The model under review builds one solid part; all positions refer to its coordinate system, in mm. A direction names the side the tool comes from. Coordinates: 2 decimals unless noted, no trailing zeros. Loops run counter-clockwise (first coordinate to the right, second up) from the corner with the lowest first, then second, coordinate; pieces in that order, holes last. Notation, with made-up numbers: M 69.5,89.5 L 111.5,89.5 A22 cw 111.5,111.5 Z; hole C -2.75,47 d10. An arc over 180 degrees is marked long. Use one line per item in the form item = value.
Autodesk Fusion 360 part; units mm, degrees
sketch "スケッチ1" plane through (0, 0, 0) normal (0, 0, 1) x (1, 0, 0)
  circle A0 centre (0, 0) radius 10
  line L0 (0, 10) -> (12, 10)
  line L1 (12, 10) -> (12, 20)
  line L2 (12, 20) -> (27, 20)
  line L3 (27, 20) -> (27, 13)
  line L4 (27, 13) -> (23, 13)
  line L5 (23, 13) -> (23, 16)
  line L6 (23, 16) -> (19, 16)
  line L7 (19, 16) -> (19, -22)
  line L8 (19, -22) -> (12, -22)
  line L9 (12, -22) -> (12, -10)
  line L10 (12, -10) -> (0, -10)
  line L11 (0, -7) -> (0, 7)
  line L12 (19, -7) -> (14, -7)
  line L13 (14, -7) -> (14, 7)
  line L14 (14, 7) -> (19, 7)
  point P0 (14, 0)
  dimension "d1" = 20
  dimension "d2" = 12
  dimension "d4" = 4
  dimension "d5" = 4
  dimension "d6" = 7
  dimension "d8" = 4
  dimension "d9" = 3
  dimension "d19" = 14
  dimension "d29" = 13
  dimension "d30" = 22
  dimension "d31" = 5
  dimension "d32" = 14
extrude "押し出し1" add sketch "スケッチ1" along normal blind 8 contours A0 | A0 L0 L1 L2 L3 L4 L5 L6 L7 L8 L9 L10 L12 L13 L14
sketch "スケッチ2" plane through (0, 0, 8) normal (0, 0, 1) x (-1, 0, 0)
  arc A0 (0, -10) -> (0, 10) centre (0, 0) ccw
  line L0 (0, 10) -> (-12, 10)
  line L1 (-12, 10) -> (-12, 22)
  line L2 (-12, 22) -> (-19, 22)
  line L3 (-19, -7) -> (-19, -16)
  line L4 (-19, -16) -> (-23, -16)
  line L5 (-23, -16) -> (-23, -13)
  line L6 (-23, -13) -> (-27, -13)
  line L7 (-27, -13) -> (-27, -20)
  line L8 (-27, -20) -> (-12, -20)
  line L9 (-12, -20) -> (-12, -10)
  line L10 (-12, -10) -> (0, -10)
  circle A1 centre (0, 0) radius 10
  line L11 (-19, 7) -> (-14, 7)
  line L12 (-14, 7) -> (-14, -7)
  line L13 (-14, -7) -> (-19, -7)
  line L14 (-19, 22) -> (-19, 7)
extrude "押し出し2" add sketch "スケッチ2" along normal blind 1.5 contours A0 A1
hole "穴1" at (0, 7, 0) at (0, -7, 0) direction (0, 0, 1) diameter 3.2 end through all
hole "穴3" at (0, 0, 0) direction (0, 0, 1) diameter 8 end through all
sketch "スケッチ3" plane through (0, -10, 0) normal (0, -1, 0) x (1, 0, 0)
  line L0 (0, 0) -> (12, 0)
  line L1 (12, 0) -> (12, 8)
  line L2 (12, 8) -> (0, 8)
  line L3 (0, 8) -> (0, 0)
  line L4 (10, 0) -> (4, 4.5)
  line L5 (4, 4.5) -> (-15, 4.5)
  line L6 (-15, 4.5) -> (-15, 0)
  line L7 (-15, 0) -> (10, 0)
  dimension "d20" = 10
  dimension "d21" = 15
  dimension "d22" = 6
  dimension "d23" = 4.5
extrude "押し出し3" cut sketch "スケッチ3" against normal through all contours L0 L3 L4 L5 L7 | L3 L5 L6 L7
sketch "スケッチ4" plane through (19, 0, 0) normal (1, 0, 0) x (0, 1, 0)
  line L0 (-22, 0) -> (-7, 0)
  line L1 (16, 0) -> (16, 8)
  line L2 (-7, 8) -> (-22, 8)
  line L3 (-22, 8) -> (-22, 0)
  line L4 (-22, 4) -> (-18, 4)
  line L5 (-7, 0) -> (-7, 8)
  line L6 (7, 0) -> (16, 0)
  line L7 (16, 8) -> (7, 8)
  line L8 (7, 8) -> (7, 0)
  dimension "d25" = 4
hole "穴2" at (19, -18, 4) direction (-1, 0, 0) diameter 3 depth 11 tip angle 118
thread "ねじ1"
chamfer "面取り1" distance 1 angle 45 1 edges at (23, 13, 4)
fillet "フィレット1" radius 4 4 edges at (12, 10, 4) (12, -10, 4) (14, -7, 4) (14, 7, 4)
1. Add section D-D (y = 17). State the section outline as (x, z) points.
Response values:
outline = M 12,0 L 27,0 L 27,8 L 12,8 Z
2. Insertion check: P1, Ø0.6, axis at y = 14.5, z = 4.5, coming from the -X side; P2, Ø8, axis at x = 15.5, y = -6, coming from the +Z side; P3, Ø5, axis at x = -4, z = 6.5, coming from the +Y side; P4, Ø3.5, axis at x = 0, y = -7, coming from the +Z side. Each pin has a flat end and moves straight along its axis. Give the tip position at first contact, or say it passes through.
Response values:
P1 = 12
P2 = 8
P3 = 9.89
P4 = 9.5
3. Wall thickness on line 1 along Y through (x, z) = (0, 6.35); line 2 along Z through (x, y) = (13.5, -18); line 3 along Y through (x, z) = (7.5, 2.5): over which ranges is each line inside the solid? List them lowest first. Write a range as from..to.
Response values:
line_1 = -10..-8.6, -5.4..-4, 4..5.4, 8.6..10
line_2 = 0..2.5, 5.5..8
line_3 = -10..10
4. The part is to be moulded in two halves that separate along X. For faces 1 (the face through (4, 10, 5)), 2 (the face through (3.905, -0.867, 7.035)), 3 (the face through (10.797, 11.141, 4.056)), 4 (the face through (23.5, 13.5, 3.9)), say which applies: pulls with the +X half, pulls with the -X half, needs draft (parallel to the pull), parting line crosses it, or undercut.
Response values:
face_1 = needs draft
face_2 = undercut
face_3 = pulls with the -X half
face_4 = undercut
5. Machinability: for faces 5 (the face through (21, 16, 4)), 6 (the face through (-4.5, -0.1, 4.5)), 7 (the face through (19, -14, 4)), 8 (the face through (18.5, -7, 3.9)), which of the approach directions +Z, -Z, +X, -X, +Y, -Y give a long, thin tool a straight path to every point of the face, cutting with its end or side? Answer none if there is none.
Response values:
face_5 = +Z, -Z, -Y
face_6 = -Z, -X, +Y, -Y
face_7 = +Z, -Z, +X, -Y
face_8 = +Z, -Z, +X
6. Add section B-B (z = 4). State the section outline as (x, y) points, then the cut area to 3 significant figures.
Response values:
outline = M 4.67,-10 L 8,-10 A4 cw 12,-14 L 12,-16.5 L 19,-16.5 L 19,-7 L 18,-7 A4 cw 14,-3 L 14,3 A4 cw 18,7 L 19,7 L 19,16 L 23,16 L 23,14 L 24,13 L 27,13 L 27,20 L 12,20 L 12,14 A4 cw 8,10 L 4.67,10 Z; M 12,-22 L 19,-22 L 19,-19.5 L 12,-19.5 Z
area = 407 mm^2
7. Add section A-A (x = 18.5). State the section outline as (y, z) points.
Response values:
outline = M -22,0 L -7,0 L -7,8 L -22,8 Z; M 7,0 L 20,0 L 20,8 L 7,8 Z; hole C -18,4 d3
